Read the model definition and answer for the solid it produces. Units are mm, in the model's axes. Face numbers are marked on the shaded views. A direction names the side the tool comes from. Coordinates: 2 decimals unless noted, no trailing zeros. Write each loop counter-clockwise with the first axis right and the second up, starting at its lowest first coordinate (ties: lowest second). Pieces come first, ordered by that corner, then holes.
Item 1: A tool of negligible diameter and unlimited length cuts with its end or side. For the marked faces 4 and 5, from which of +Z, -Z, +X, -X, +Y, -Y can it reach the whole face along a straight path? Write none if from no direction.
Item 2: Straight lines are drawn through the part: probe 1 along Z at (x, y) = (-20, -7.5); probe 2 along Y at (x, z) = (-22.75, -0.25); probe 3 along Y at (x, z) = (-14.5, -4.75). For each, find the intervals that lie inside material, in ascending order.
Item 3: Each of these flat-tipped pins is pushed along its axis until it touches: P1, Ø4.5, axis at x = -16.5, z = -2, coming from the -Y side; P2, Ø6, axis at x = -9, z = -3, coming from the +Y side; P3, Ø5, axis at y = -9.5, z = 1.5, coming from the -X side. Where does it stop, or does it pass through?
Item 4: Determine the mould class of the marked faces 1, 2 and 3 for opening direction Z: released by +Z, released by -Z, zero draft, split by the parting line, or undercut.
Item 5: Section B-B (x = -6) is taken. Give the vertices of the cut face in (y, z).
Item 6: Section C-C (z = -1) is taken. Give the vertices of the cut face in (x, y).
Item 7: Section D-D (y = -7) is taken. Give the vertices of the cut face in (x, z).
Item 8: Section A-A (y = -3.5) is taken. Give the vertices of the cut face in (x, z).
from build123d import *

# Parameters (mm, degrees)
BOSS_EXTRUDE1_DEPTH = 3
SKETCH2_W           = 28
SKETCH2_H           = 2
BOSS_EXTRUDE2_DEPTH = 4
BOSS_EXTRUDE3_START = 3
BOSS_EXTRUDE3_DEPTH = 3
SKETCH4_W           = 28
SKETCH4_H           = 5.276937717
CUT_EXTRUDE1_DEPTH  = 1.5


with BuildPart() as part:
    # Sketch1 → Boss-Extrude1 (new body)
    with BuildSketch(Plane.XY):
        with BuildLine():
            Line((-26.074492775, 2.891966759), (1.925507225, 2.891966759))
            Line((1.925507225, 2.891966759), (1.925507225, -5.108033241))
            ThreePointArc((1.925507225, -5.108033241), (-12.074492775, -19.108033241), (-26.074492775, -5.108033241))
            Line((-26.074492775, -5.108033241), (-26.074492775, 2.891966759))
        make_face()
    extrude(amount=BOSS_EXTRUDE1_DEPTH)

    # Sketch2 → Boss-Extrude2 (add)
    with BuildSketch(Plane(origin=(0, 0, 0), x_dir=(-1, 0, 0), z_dir=(0, 0, -1))):
        with Locations((12.074492775, 1.891966759)):
            Rectangle(SKETCH2_W, SKETCH2_H)
    extrude(amount=BOSS_EXTRUDE2_DEPTH)

    # Sketch3 → Boss-Extrude3 (add)
    with BuildSketch(Plane(origin=(0, 0, -4), x_dir=(-1, 0, 0), z_dir=(0, 0, -1)).offset(BOSS_EXTRUDE3_START)):
        with BuildLine():
            Line((-1.925507225, 2.891966759), (26.074492775, 2.891966759))
            Line((26.074492775, 2.891966759), (26.074492775, -5.108033241))
            ThreePointArc((26.074492775, -5.108033241), (12.074492775, -19.108033241), (-1.925507225, -5.108033241))
            Line((-1.925507225, -5.108033241), (-1.925507225, 2.891966759))
        make_face()
    extrude(amount=-BOSS_EXTRUDE3_DEPTH)

    # Sketch4 → Cut-Extrude1 (cut)
    with BuildSketch(Plane(origin=(0, 2.891966759, 0), x_dir=(1, 0, 0), z_dir=(0, 1, 0))):
        with Locations((-12.074492775, 1.861531141)):
            Rectangle(SKETCH4_W, SKETCH4_H)
    extrude(amount=-CUT_EXTRUDE1_DEPTH, mode=Mode.SUBTRACT)


solid = part.part
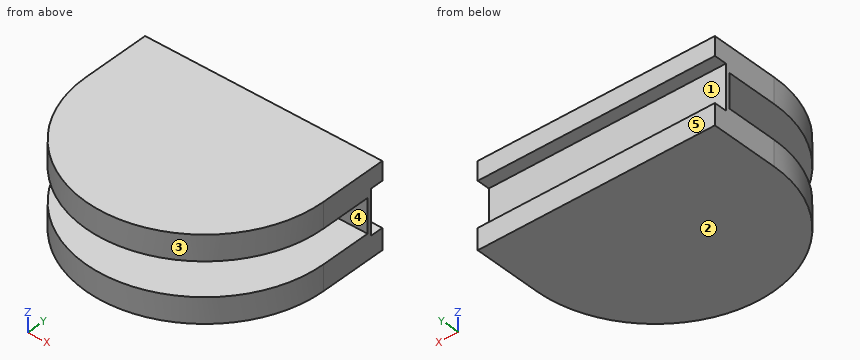
Established:
1. face 4: +X, -X, -Y
1. face 5: +Z, -Z, +X, -X, +Y
2. probe 1: z = -7 to -4, 0 to 3
2. probe 2: y = 0.89 to 1.39
2. probe 3: y = -18.9 to 2.89
3. P1: stops at y = -18.69
3. P2: stops at y = 2.89
3. P3: stops at x = -25.95
4. face 1: undercut
4. face 2: released by -Z
4. face 3: zero draft
5. outline: (-17.72, -7) - (2.89, -7) - (2.89, -4.5) - (1.39, -4.5) - (1.39, 0.78) - (2.89, 0.78) - (2.89, 3) - (-17.72, 3) - (-17.72, 0) - (0.89, 0) - (0.89, -4) - (-17.72, -4) - close
6. outline: (-26.07, 0.89) - (1.93, 0.89) - (1.93, 1.39) - (-26.07, 1.39) - close
7. outline: (-25.95, -7) - (1.8, -7) - (1.8, -4) - (-25.95, -4) - close; (-25.95, 0) - (1.8, 0) - (1.8, 3) - (-25.95, 3) - close
8. outline: (-26.07, -7) - (1.93, -7) - (1.93, -4) - (-26.07, -4) - close; (-26.07, 0) - (1.93, 0) - (1.93, 3) - (-26.07, 3) - close
